For this review, take the finished solid that the model builds, in its own axes (mm). Face numbers are marked on the shaded views. A direction names the side the tool comes from. Round coordinates to 2 decimals unless told otherwise and drop trailing zeros. Order: outer loops, then holes, each group sorted by start corner. A loop starts at its lowest first (then second) coordinate and runs counter-clockwise, first axis right, second up.
```python
from build123d import *

# Parameters (mm, degrees)
SKETCH1_W           = 74.8
SKETCH1_H           = 40
BOSS_EXTRUDE1_DEPTH = 10
BOSS_EXTRUDE2_DEPTH = 5
BOSS_EXTRUDE3_DEPTH = 84.8
SKETCH4_W           = 77.196671852
SKETCH4_H           = 40
CUT_EXTRUDE1_DEPTH  = 59


with BuildPart() as part:
    # Sketch1 → Boss-Extrude1 (new body)
    with BuildSketch(Plane(origin=(0, 0, 0), x_dir=(1, 0, 0), z_dir=(0, 1, 0))):
        Rectangle(SKETCH1_W, SKETCH1_H)
    extrude(amount=BOSS_EXTRUDE1_DEPTH)

    # Sketch2 → Boss-Extrude2 (add)
    # profile 1 of 2: a face of its own
    with BuildSketch(Plane(origin=(37.4, 0, 0), x_dir=(0, 0, -1), z_dir=(1, 0, 0))):
        with BuildLine():
            Line((7.5, 0), (-7.5, 0))
            Line((-7.5, 0), (-7.5, -6))
            Line((-7.5, -6), (-5.665, -6))
            ThreePointArc((-5.665, -6), (0, -11.665), (5.665, -6))
            Line((5.665, -6), (7.5, -6))
            Line((7.5, -6), (7.5, 0))
        make_face()
        with BuildLine():
            ThreePointArc((2.82, -6), (0, -8.82), (-2.82, -6))
            ThreePointArc((-2.82, -6), (0, -3.18), (2.82, -6))
        make_face(mode=Mode.SUBTRACT)
    # profile 2 of 2: a face of its own
    with BuildSketch(Plane(origin=(37.4, 0, 0), x_dir=(0, 0, -1), z_dir=(1, 0, 0))):
        Polygon((-20, 0), (-7.5, 0), (7.5, 0), (20, 0), (20, 10), (-20, 10), align=None)
    boss_extrude2 = extrude(amount=BOSS_EXTRUDE2_DEPTH)

    # Mirror1: Boss-Extrude2 across plane
    add(boss_extrude2.mirror(Plane(origin=(0, 0, 0), x_dir=(0, 0, 1), z_dir=(1, 0, 0))))

    # Sketch3 → Boss-Extrude3 (add)
    with BuildSketch(Plane.ZY.offset(42.4)):
        with BuildLine():
            Line((-3.838227356, 14.8), (-3.838227356, 10))
            Line((-3.838227356, 10), (3.838227356, 10))
            Line((3.838227356, 10), (3.838227356, 14.8))
            Line((3.838227356, 14.8), (6.838227356, 14.8))
            Line((6.838227356, 14.8), (6.838227356, 14.3))
            ThreePointArc((6.838227356, 14.3), (7.131120575, 13.592893219), (7.838227356, 13.3))
            Line((7.838227356, 13.3), (9.438227356, 13.3))
            Line((9.438227356, 13.3), (9.438227356, 14.8))
            Line((9.438227356, 14.8), (9.438227356, 18.08))
            Line((9.438227356, 18.08), (5.3521045, 21.88))
            Line((5.3521045, 21.88), (-5.3521045, 21.88))
            Line((-5.3521045, 21.88), (-9.438227356, 18.08))
            Line((-9.438227356, 18.08), (-9.438227356, 14.8))
            Line((-9.438227356, 14.8), (-9.438227356, 13.3))
            Line((-9.438227356, 13.3), (-7.838227356, 13.3))
            ThreePointArc((-7.838227356, 13.3), (-7.131120575, 13.592893219), (-6.838227356, 14.3))
            Line((-6.838227356, 14.3), (-6.838227356, 14.8))
            Line((-6.838227356, 14.8), (-3.838227356, 14.8))
        make_face()
    extrude(amount=-BOSS_EXTRUDE3_DEPTH)

    # Sketch4 → Cut-Extrude1 (cut)
    with BuildSketch(Plane(origin=(0, 21.88, 0), x_dir=(1, 0, 0), z_dir=(0, 1, 0))):
        with Locations((3.801664074, 0)):
            Rectangle(SKETCH4_W, SKETCH4_H)
    extrude(amount=-CUT_EXTRUDE1_DEPTH, mode=Mode.SUBTRACT)


solid = part.part
```
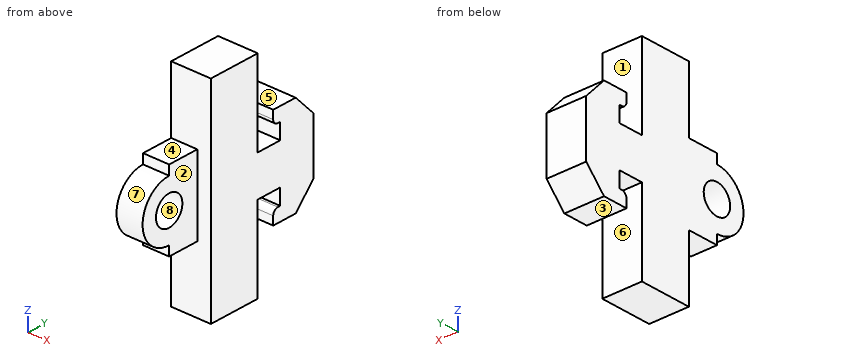
Q1. Take a section at A-A, the plane z = 0. State the section outline as (x, y) points (3 decimals).
Q2. Take a section at B-B, the plane x = -41. State the section outline as (y, z) points (3 decimals).
Q3. Mouldability with a two-part tool opening along Y and no side actions: class the marked faces 5, 6, 7 and 8 as +Y half, -Y half, draft (parallel to the pull), parting line (faces both ways), or undercut.
Q4. Tool access review of the marked faces 1, 2, 3 and 4: name each direction out of +Z, -Z, +X, -X, +Y, -Y from which nothing blocks a thin tool from reaching the whole face with its end or side.
Q5. Take a section at C-C, the plane x = -36. State the section outline as (y, z) points.
Q6. Wall thickness on line 1 (Y direction, x = -40.2, z = 0) (3 decimals); line 2 (Y direction, x = -36.5, z = -10); line 3 (X direction, y = -4.5, z = -3): over which ranges is each line inside the solid? List them lowest first.
Q7. Take a section at D-D, the plane z = -10. State the section outline as (x, y) points.
Q8. Clearance check with flat-ended pins moving along their axes: pin 1 (1.5 mm diameter, centred on x = -41, y = -3.5, fed in from -Z); pin 2 (4 mm diameter, centred on x = -41, z = 5.5, fed in from -Y); pin 3 (2.5 mm diameter, centred on x = -40, y = 15.5, fed in from -Z). State where each tip first meets the part, or that it passes through.
Working result:
1. outline: (-42.4, -11.665) - (-37.4, -11.665) - (-37.4, -8.82) - (-42.4, -8.82) - close; (-42.4, -3.18) - (-37.4, -3.18) - (-37.4, 0) - (-34.797, 0) - (-34.797, 21.88) - (-42.4, 21.88) - close
2. outline: (-6, -7.5) - (0, -7.5) - (0, -20) - (10, -20) - (10, -3.838) - (14.8, -3.838) - (14.8, -6.838) - (14.3, -6.838) arc R1 ccw to (13.3, -7.838) - (13.3, -9.438) - (18.08, -9.438) - (21.88, -5.352) - (21.88, 5.352) - (18.08, 9.438) - (13.3, 9.438) - (13.3, 7.838) arc R1 ccw to (14.3, 6.838) - (14.8, 6.838) - (14.8, 3.838) - (10, 3.838) - (10, 20) - (0, 20) - (0, 7.5) - (-6, 7.5) - (-6, 5.665) arc R5.665 ccw to (-6, -5.665) - close; hole circle Ø5.64 at (-6, 0)
3. face 5: draft
3. face 6: undercut
3. face 7: -Y half
3. face 8: undercut
4. face 1: +Z, +X, -X
4. face 2: +Z, -Z, +X, -Y
4. face 3: -Z, +X, -X, +Y
4. face 4: +Z, +X, -X, -Y
5. outline: (0, -20) - (10, -20) - (10, -3.84) - (14.8, -3.84) - (14.8, -6.84) - (14.3, -6.84) arc R1 ccw to (13.3, -7.84) - (13.3, -9.44) - (18.08, -9.44) - (21.88, -5.35) - (21.88, 5.35) - (18.08, 9.44) - (13.3, 9.44) - (13.3, 7.84) arc R1 ccw to (14.3, 6.84) - (14.8, 6.84) - (14.8, 3.84) - (10, 3.84) - (10, 20) - (0, 20) - close
6. line 1: y = -11.665 to -8.82, -3.18 to 21.88
6. line 2: y = 0 to 10
6. line 3: x = -42.4 to -37.4
7. outline: (-42.4, 0) - (-34.8, 0) - (-34.8, 10) - (-42.4, 10) - close
8. pin 1: stops at z = -7.5
8. pin 2: stops at y = -10.45
8. pin 3: stops at z = -9.44
